For this review, take the finished solid that the model builds, in its own axes (mm). A direction names the side the tool comes from. Round coordinates to 2 decimals unless told otherwise and drop trailing zeros. Write each loop counter-clockwise with the first axis right and the second up, starting at its lowest first coordinate (ties: lowest second). Pieces come first, ordered by that corner, then holes. Notation, with made-up numbers: (7.25, 38) -> (28.25, 38) arc R28 ccw to (28.25, 66) -> close; hole circle Ø10 at (-25.5, 89.25). An arc over 180 degrees is marked (long way). Answer as CSV lines item,"result". Start each with the question number.
Item 1: Take a section at C-C on z = 5.25. Give the boundary of the cut face in (x, y).
Item 2: Machinability: for faces 1 (the cylindrical face through (-7.15, 22.63, 1.48)), 2 (the cylindrical face through (-13.986, 0.616, 10.274)), which of the approach directions +Z, -Z, +X, -X, +Y, -Y give a long, thin tool a straight path to every point of the face, cutting with its end or side? Answer none if there is none.
Item 3: For pin 1 Ø2 at (x, z) = (-7, 10) entering from +Y; pin 2 Ø4 at (x, y) = (-3.5, 9) entering from +Z; pin 3 Ø8 at (x, y) = (-26, 0) entering from +Z; pin 4 Ø1 at (x, y) = (1.5, -16) entering from +Z, all flat-tipped, find the tip position at first contact; note any pin that passes through.
Item 4: Mouldability with a two-part tool opening along X and no side actions: class faces 3 (the cylindrical face through (-2.38, -10.74, 6.08)), 4 (the cylindrical face through (32, 0, 1)), 5 (the flat face through (0, 15, 0)) as +X half, -X half, draft (parallel to the pull), parting line (faces both ways), or undercut.
Item 5: Wall thickness on probe 1 along Y at (x, z) = (-26, 0.8); probe 2 along Y at (x, z) = (0, 9.5); probe 3 along Y at (x, z) = (1.5, 2.25): over which ranges is each line inside the solid? List them lowest first. Write a range as from..to.
Item 6: Take a section at A-A on y = 0. Count the separate pieces of the cut face and the enclosed holes in it, then the cut area to 3 significant figures.
```python
from build123d import *

# Parameters (mm, degrees)
PAD_DEPTH             = 12
POLARPATTERN_COUNT    = 4
SKETCH003_R           = 11
POCKET_DEPTH          = 12.001
SKETCH004_R           = 2.5
POCKET001_DEPTH       = 185.604396
POLARPATTERN001_COUNT = 4


with BuildPart() as part:
    # Sketch → Pad (new body)
    with BuildSketch(Plane.XY):
        with BuildLine():
            ThreePointArc((15.909903, 15.909903), (13.086202, 18.303041), (9.908356, 20.200854))
            ThreePointArc((5.995813, 26.224112), (7.120676, 22.672423), (9.908356, 20.200854))
            ThreePointArc((5.995813, 26.224112), (0, 32), (-5.995813, 26.224112))
            ThreePointArc((-9.908356, 20.200854), (-7.120676, 22.672423), (-5.995813, 26.224112))
            ThreePointArc((-9.908356, 20.200854), (-13.086202, 18.303041), (-15.909903, 15.909903))
            Line((-15.909903, 15.909903), (0, 0))
            Line((0, 0), (15.909903, 15.909903))
        make_face()
    pad = extrude(amount=PAD_DEPTH)

    # PolarPattern: Pad ×4 about axis
    polarpattern_axis = Axis((0, 0, 0), (0, 0, 1))
    for i in range(1, POLARPATTERN_COUNT):
        add(pad.rotate(polarpattern_axis, i * 360 / POLARPATTERN_COUNT))

    # SubtractivePipe: sweep along a path in Sketch002
    with BuildLine(Plane.XY.offset(12)) as subtractivepipe_path:
        CenterArc((0, 0), 14, 0, 360)
    # Sketch001 → SubtractivePipe (sweep, cut)
    with BuildSketch(Plane.YZ):
        with BuildLine():
            Line((-14, 12), (-32, 12))
            Line((-32, 12), (-32, 3))
            Line((-32, 3), (-18.5, 3))
            ThreePointArc((-18.5, 3), (-17.43934, 3.43934), (-17, 4.5))
            Line((-17, 4.5), (-17, 8.5))
            Line((-17, 8.5), (-14, 8.5))
            Line((-14, 8.5), (-14, 12))
        make_face()
    sweep(path=subtractivepipe_path.line, mode=Mode.SUBTRACT)

    # Sketch003 (on Face31 of SubtractivePipe) → Pocket (cut, through all)
    with BuildSketch(Plane.XY.offset(12)):
        Circle(SKETCH003_R)
    extrude(amount=-POCKET_DEPTH, mode=Mode.SUBTRACT)

    # Sketch004 (on Face4 of Pocket) → Pocket001 (cut, through all)
    with BuildSketch(Plane.XY.offset(3)):
        with Locations((0, 26)):
            Circle(SKETCH004_R)
    pocket001 = extrude(amount=-POCKET001_DEPTH, mode=Mode.SUBTRACT)

    # PolarPattern001: Pocket001 ×4 about axis
    polarpattern001_axis = Axis((0, 0, 3), (0, 0, 1))
    for i in range(1, POLARPATTERN001_COUNT):
        add(pocket001.rotate(polarpattern001_axis, i * 360 / POLARPATTERN001_COUNT), mode=Mode.SUBTRACT)


solid = part.part
```
Output values:
1,outline,"circle Ø34 at (0, 0); hole circle Ø22 at (0, 0)"
2,face 1,"+Z, -Z, -X, +Y"
2,face 2,"+Z"
3,pin 1,"stops at y = 12.65"
3,pin 2,"stops at z = 12"
3,pin 3,"stops at z = 3"
3,pin 4,"stops at z = 8.5"
4,face 3,"undercut"
4,face 4,"+X half"
4,face 5,"draft"
5,probe 1,"y = -6.01..-2.5, 2.5..6.01"
5,probe 2,"y = -14..-11, 11..14"
5,probe 3,"y = -31.81..-28, -24..-10.9, 10.9..24, 28..31.81"
6,separate pieces,"4"
6,enclosed holes,"0"
6,area,"184 mm^2"
